```python
from build123d import *

# Parameters (mm, degrees)
EXTRUDE_1_DEPTH     = 4
SKETCH_3_R          = 2.5
CUT_EXTRUDE_1_DEPTH = 24
SKETCH_4_R          = 1.525
CUT_EXTRUDE_2_DEPTH = 5
SKETCH_5_R          = 2.5
CUT_EXTRUDE_3_DEPTH = 5
FILLET_1_R          = 5
SKETCH_6_R          = 1.6
SKETCH_6_R_2        = 10
CUT_EXTRUDE_4_DEPTH = 10
SKETCH_7_R          = 17.5
SKETCH_7_R_2        = 10
SKETCH_7_R_3        = 1.6
EXTRUDE_2_DEPTH     = 4
FILLET_2_R          = 5
EXTRUDE_START       = -4
SKETCH_8_R          = 2.5
EXTRUDE_3_DEPTH     = 4
SKETCH_9_R          = 2.5
EXTRUDE_4_DEPTH     = 4


with BuildPart() as part:
    # 草图1 → 凸台-拉伸1 (new body)
    with BuildSketch(Plane.XY):
        with BuildLine():
            Line((6, -7.365459931), (6, -45))
            ThreePointArc((6, -45), (0, -51), (-6, -45))
            Line((-6, -45), (-6, -7.365459931))
            ThreePointArc((-6, -7.365459931), (0, 9.5), (6, -7.365459931))
        make_face()
    extrude(amount=EXTRUDE_1_DEPTH)

    # 草图3 → 切除-拉伸1 (cut)
    with BuildSketch(Plane.XY.offset(4)):
        with Locations((0, -45)):
            Circle(SKETCH_3_R)
    extrude(amount=-CUT_EXTRUDE_1_DEPTH, mode=Mode.SUBTRACT)

    # 草图4 → 切除-拉伸2 (cut)
    with BuildSketch(Plane.XY.offset(4)):
        with Locations((0, 6.25)):
            Circle(SKETCH_4_R)
        with Locations((0, -6.25)):
            Circle(SKETCH_4_R)
    extrude(amount=-CUT_EXTRUDE_2_DEPTH, mode=Mode.SUBTRACT)

    # 草图5 → 切除-拉伸3 (cut)
    with BuildSketch(Plane.XY.offset(4)):
        Circle(SKETCH_5_R)
    extrude(amount=-CUT_EXTRUDE_3_DEPTH, mode=Mode.SUBTRACT)

    # 圆角1
    fillet_1_edges = [part.edges().sort_by_distance(p)[0] for p in [
        (-6, -7.365459931, 2),
        (6, -7.365459931, 2),
    ]]
    fillet(fillet_1_edges, radius=FILLET_1_R)

    # 草图6 → 切除-拉伸4 (cut)
    with BuildSketch(Plane.XY.offset(4)):
        with Locations((0, -13.5)):
            Circle(SKETCH_6_R)
        Circle(SKETCH_6_R_2)
    extrude(amount=-CUT_EXTRUDE_4_DEPTH, mode=Mode.SUBTRACT)

    # 草图7 → 凸台-拉伸2 (add)
    with BuildSketch(Plane.XY.offset(4)):
        Circle(SKETCH_7_R)
        Circle(SKETCH_7_R_2, mode=Mode.SUBTRACT)
        with Locations((11.691342951, 6.75)):
            Circle(SKETCH_7_R_3, mode=Mode.SUBTRACT)
        with Locations((-11.691342951, 6.75)):
            Circle(SKETCH_7_R_3, mode=Mode.SUBTRACT)
        with Locations((0, -13.5)):
            Circle(SKETCH_7_R_3, mode=Mode.SUBTRACT)
    extrude(amount=-EXTRUDE_2_DEPTH)

    # 圆角2
    fillet_2_edges = [part.edges().sort_by_distance(p)[0] for p in [
        (6, -16.439282223, 2),
        (-6, -16.439282223, 2),
    ]]
    fillet(fillet_2_edges, radius=FILLET_2_R)

    # 草图8 → 凸台-拉伸3 (add)
    # profile 1 of 4: a face of its own
    with BuildSketch(Plane.XY.offset(4).offset(EXTRUDE_START)):
        with BuildLine():
            ThreePointArc((3.427769437, -49.924469178), (5.318205366, -52.071044966), (6, -54.848938357))
            Line((6, -54.848938357), (6, -45))
            ThreePointArc((6, -45), (5.318205366, -47.777893391), (3.427769437, -49.924469178))
        make_face()
    # profile 2 of 4: a face of its own
    with BuildSketch(Plane.XY.offset(4).offset(EXTRUDE_START)):
        with BuildLine():
            Line((-6, -45), (-6, -54.848938357))
            ThreePointArc((-6, -54.848938357), (-5.318205366, -52.071044966), (-3.427769437, -49.924469178))
            ThreePointArc((-3.427769437, -49.924469178), (-5.318205366, -47.777893391), (-6, -45))
        make_face()
    # profile 3 of 4: a face of its own
    with BuildSketch(Plane.XY.offset(4).offset(EXTRUDE_START)):
        with BuildLine():
            Line((-6, -40), (-6, -45))
            ThreePointArc((-6, -45), (-5.318205366, -47.777893391), (-3.427769437, -49.924469178))
            ThreePointArc((-3.427769437, -49.924469178), (0, -48.848938357), (3.427769437, -49.924469178))
            ThreePointArc((3.427769437, -49.924469178), (5.318205366, -47.777893391), (6, -45))
            Line((6, -45), (6, -40))
            Line((6, -40), (-6, -40))
        make_face()
        with Locations((0, -45)):
            Circle(SKETCH_8_R, mode=Mode.SUBTRACT)
    # profile 4 of 4: a face of its own
    with BuildSketch(Plane.XY.offset(4).offset(EXTRUDE_START)):
        with BuildLine():
            ThreePointArc((-3.427769437, -49.924469178), (-5.318205366, -52.071044966), (-6, -54.848938357))
            ThreePointArc((-6, -54.848938357), (0, -60.848938357), (6, -54.848938357))
            ThreePointArc((6, -54.848938357), (5.318205366, -52.071044966), (3.427769437, -49.924469178))
            ThreePointArc((3.427769437, -49.924469178), (0, -51), (-3.427769437, -49.924469178))
        make_face()
        with Locations((0, -54.848938357)):
            Circle(SKETCH_8_R, mode=Mode.SUBTRACT)
    extrude(amount=EXTRUDE_3_DEPTH)

    # 草图9 → 凸台-拉伸4 (add)
    with BuildSketch(Plane.XY.offset(4)):
        with Locations((0, -45)):
            Circle(SKETCH_9_R)
    extrude(amount=-EXTRUDE_4_DEPTH)


solid = part.part
```
Input: part model. Units: mm. Frame: model coordinates. A direction names the side the tool comes from. Round coordinates to 2 decimals unless told otherwise and drop trailing zeros. Write each loop counter-clockwise with the first axis right and the second up, starting at its lowest first coordinate (ties: lowest second). Pieces come first, ordered by that corner, then holes. Notation, with made-up numbers: (7, -5.75) -> (60, -5.75) arc R17 cw to (60, 19.25) -> close; hole circle Ø7 at (-23, 40). An arc over 180 degrees is marked (long way). Answer as CSV lines item,"result".
1. Ray query, L1, parallel to Y at x = 0, z = 1.2; L2, parallel to Y at x = 2, z = 1.85; L3, parallel to X at y = -13, z = 1.85. Return the intervals inside material, ascending. Write a range as [from, to].
Geometry says:
L1,"y = [-60.85, -57.35], [-52.35, -15.1], [-11.9, -10], [10, 17.5]"
L2,"y = [-60.51, -56.35], [-53.35, -9.8], [9.8, 17.39]"
L3,"x = [-11.72, -1.52], [1.52, 11.72]"
2. Mould query, pull axis X, two halves, no side actions, for faces 3 (the flat face through (-6, -37, 2)), 4 (the cylindrical face through (-0.5, -57.3, 2)), 5 (the cylindrical face through (11.3, 5.2, 2)), 6 (the cylindrical face through (6.705, -17.068, 2.028)). Classes: +X half, -X half, draft (parallel to the pull), parting line (faces both ways), or undercut.
Geometry says:
face 3,"-X half"
face 4,"undercut"
face 5,"undercut"
face 6,"+X half"
3. Contact query for flat-ended pins moving along their axis: P1, Ø1.2, axis at y = -35, z = 1.5, coming from the -X side; P2, Ø1.2, axis at y = -33.5, z = 2, coming from the +X side; P3, Ø1.5, axis at y = -3, z = 3.5, coming from the -X side. Output: stop coordinate, or through.
Geometry says:
P1,"stops at x = -6"
P2,"stops at x = 6"
P3,"stops at x = -17.35"
4. Section B-B (z = 3.1). Return the cut outline in (x, y), plus the area to 3 significant figures.
Geometry says:
outline,"(-8.56, -15.27) arc R5 cw to (-6, -19.63) -> (-6, -54.85) arc R6 ccw to (6, -54.85) -> (6, -19.63) arc R5 cw to (8.56, -15.27) arc R17.5 ccw (long way) to start; hole circle Ø3.2 at (-11.69, 6.75); hole circle Ø20 at (0, 0); hole circle Ø5 at (0, -54.85); hole circle Ø3.2 at (0, -13.5); hole circle Ø3.2 at (11.69, 6.75)"
area,"1,120 mm^2"
5. Section D-D (x = -12). Return the cut outline in (y, z), plus the area to 3 significant figures.
Geometry says:
outline,"(-12.74, 0) -> (5.18, 0) -> (5.18, 4) -> (-12.74, 4) -> close; (8.32, 0) -> (12.74, 0) -> (12.74, 4) -> (8.32, 4) -> close"
area,"89.3 mm^2"
6. Section C-C (y = 6.75). Return the cut outline in (x, z).
Geometry says:
outline,"(-16.15, 0) -> (-13.29, 0) -> (-13.29, 4) -> (-16.15, 4) -> close; (-10.09, 0) -> (-7.38, 0) -> (-7.38, 4) -> (-10.09, 4) -> close; (7.38, 0) -> (10.09, 0) -> (10.09, 4) -> (7.38, 4) -> close; (13.29, 0) -> (16.15, 0) -> (16.15, 4) -> (13.29, 4) -> close"
7. Reachability of faces 1 (the flat face through (6, -37, 2)), 2 (the cylindrical face through (0.64, 17.49, 2.03)) from +Z, -Z, +X, -X, +Y, -Y: full face, straight path, thin tool, end or side. Return the list, or none.
Geometry says:
face 1,"+Z, -Z, +X, -Y"
face 2,"+Z, -Z"
8. Section A-A (x = 0). Return the cut outline in (y, z), plus the area to 3 significant figures.
Geometry says:
outline,"(-60.85, 0) -> (-57.35, 0) -> (-57.35, 4) -> (-60.85, 4) -> close; (-52.35, 0) -> (-15.1, 0) -> (-15.1, 4) -> (-52.35, 4) -> close; (-11.9, 0) -> (-10, 0) -> (-10, 4) -> (-11.9, 4) -> close; (10, 0) -> (17.5, 0) -> (17.5, 4) -> (10, 4) -> close"
area,"201 mm^2"
